Autodesk Inventor part; units mm, degrees
ref_plane "YZ Plane" through (0, 0, 0) normal (1, 0, 0) x (0, 1, 0)
ref_plane "XZ Plane" through (0, 0, 0) normal (0, 1, 0) x (-1, 0, 0)
ref_plane "XY Plane" through (0, 0, 0) normal (0, 0, 1) x (1, 0, 0)
sketch "Sketch1" plane through (0, 0, 0) normal (1, 0, 0) x (0, 1, 0)
  circle A0 centre (-16.5288, 14.8074) radius 3.9624 construction
  circle A1 centre (-54.1655, 3.0444) radius 2.1844 construction
  circle A2 centre (-52.1252, -9.4907) radius 2.1844 construction
  circle A3 centre (-54.1655, 3.0444) radius 2.3495
  circle A4 centre (-52.1252, -9.4907) radius 2.3495
  circle A5 centre (-54.1655, 3.0444) radius 6.35
  circle A6 centre (-52.1252, -9.4907) radius 6.35
  line L0 (-60.433, 2.0242) -> (-58.3927, -10.5108)
  arc A7 (-18.8318, 15.5275) -> (-14.2258, 14.0872) centre (-16.5288, 14.8074) ccw
  line L1 (-16.5288, 14.8074) -> (-18.8318, 15.5275) construction
  line L2 (-16.5288, 14.8074) -> (-14.2258, 14.0872) construction
  arc A8 (-21.8622, 16.475) -> (-11.1955, 13.1397) centre (-16.5288, 14.8074) ccw
  line L3 (-11.1955, 13.1397) -> (-21.8622, 16.475)
  arc A9 (-11.1955, 13.1397) -> (-14.2258, 14.0872) centre (-12.6506, 13.8055) ccw
  arc A10 (-18.8318, 15.5275) -> (-21.8622, 16.475) centre (-20.287, 16.1933) ccw
  line L4 (-20.666, 17.748) -> (-55.6696, 9.2136)
  line L5 (-13.2973, 10.2485) -> (-48.4531, -14.6712)
  circle A11 centre (-26.2996, 8.7467) radius 2.3495
  point P0 (0, 0)
  point P1 (-18.8318, 15.5275)
  dimension "d0" = 4.699
  dimension "d1" = 4.699
  dimension "d4" = 12.7
  dimension "d5" = 12.7
  dimension "d6" = 2.413
  dimension "d7" = 180
  dimension "d8" = 3.175
  dimension "d9" = 1.6002
  dimension "d10" = 1.6002
  dimension "d11" = 4.699
extrude "Plate1" add sketch "Sketch1" along normal blind 1.5875 contours A5 | A5 L4 A10 A8 L5 A6 | A6 L0 A5 | A6 | A7 L3 A8
sheet face with bend "Face2" sketch "Sketch1" thickness 1.5875 toward (1, 0, 0) bend radius 1.5875 contours A10 L3 | A9 L3
bend "Bend1"
equation "\"d12\" = Thickness"
equation "\"d13\" = BendRadius"
equation "\"d14\" = BendReliefWidth"
equation "\"d16\" = MinimumRemnant"
equation "\"d15\" = BendReliefDepth"
equation "\"d17\" = TransitionRadius"
equation "\"BendRadius\" = Thickness"
equation "\"BendReliefWidth\" = Thickness"
equation "\"BendReliefDepth\" = 0.5 * Thickness"
equation "\"CornerReliefSize\" = 4 * Thickness"
equation "\"MinimumRemnant\" = 2 * Thickness"
equation "\"TransitionRadius\" = BendRadius"
equation "\"JacobiRadiusSize\" = BendRadius"
equation "\"GapSize\" = Thickness"
properties part number "hangPin"
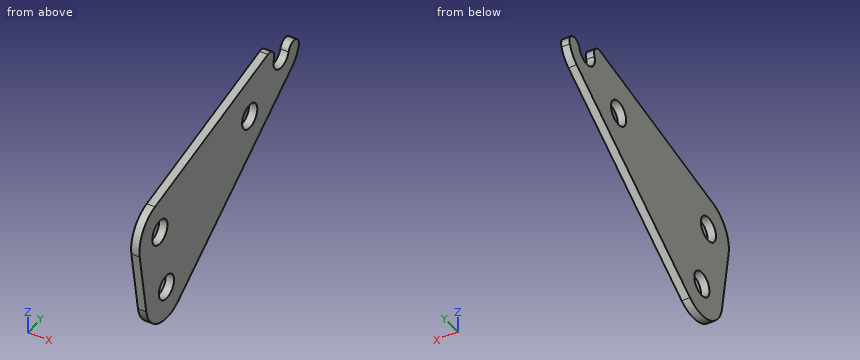
CAD build for the part. Positions are in the model's coordinates, mm. Round coordinates to 2 decimals unless told otherwise and drop trailing zeros. Loops run counter-clockwise (first coordinate to the right, second up) from the corner with the lowest first, then second, coordinate; pieces in that order, holes last. Notation, with made-up numbers: M -13.75,74.5 L 12.25,74.5 A19 ccw 12.25,111.5 Z; hole C -35,46.5 d9. An arc over 180 degrees is marked long. Return JSON: item names as keys, results as strings. Group by question number.
(1) Saw through at B-B, the plane z = -9. List the corners of the cut face in (x, y), and give its area (3 significant figures).
(2) Saw through at C-C, the plane x = 1.1. List the corners of the cut face in (y, z).
(3) Wall check: probe 1 along Z at (x, y) = (0.85, -55); probe 2 along Z at (x, y) = (1.55, -51); probe 3 along Y at (x, z) = (0.4, 0). Give the ranges that are in metal, low to high. Write a range as [from, to].
(4) Saw through at D-D, the plane y = -38. List the corners of the cut face in (x, z), and give its area (3 significant figures).
(5) Saw through at A-A, the plane y = -27. List the corners of the cut face in (x, z).
(6) Drop a flat-ended pin along its axis: P1, Ø5.5, axis at y = -26.3, z = 8.75, coming from the +X side. Give the stop position or say it passes through.
Answer list:
{
 "1": {"outline": "M 0,-58.64 L 1.59,-58.64 L 1.59,-54.42 L 0,-54.42 Z; M 0,-49.83 L 1.59,-49.83 L 1.59,-40.45 L 0,-40.45 Z", "area": "21.6 mm2"},
 "2": {"outline": "M -60.43,2.02 L -58.39,-10.51 A6.35 ccw -48.45,-14.67 L -13.3,10.25 A5.59 ccw -11.2,13.14 A1.6 ccw long -14.23,14.09 A2.41 cw -18.83,15.53 A1.6 ccw -20.67,17.75 L -55.67,9.21 A6.35 ccw Z; hole C -54.17,3.04 d4.7; hole C -52.13,-9.49 d4.7; hole C -26.3,8.75 d4.7"},
 "3": {"probe 1": "[-15.15, 0.85], [5.24, 9.38]", "probe 2": "[-15.74, -11.55], [-7.43, 10.35]", "probe 3": "[-60.1, -27.76]"},
 "4": {"outline": "M 0,-7.26 L 1.59,-7.26 L 1.59,13.52 L 0,13.52 Z", "area": "33.0 mm2"},
 "5": {"outline": "M 0,0.54 L 1.59,0.54 L 1.59,6.5 L 0,6.5 Z; M 0,10.99 L 1.59,10.99 L 1.59,16.2 L 0,16.2 Z"},
 "6": {"P1": "x = 1.59"}
}
